The drawing under review shows one solid part. Ordinate dimensions are in mm from its lowest x, y, z. A direction names the side the tool comes from. Coordinates: 2 decimals unless noted, no trailing zeros. Write each loop counter-clockwise with the first axis right and the second up, starting at its lowest first coordinate (ties: lowest second). Pieces come first, ordered by that corner, then holes. Notation, with made-up numbers: (77, 23) - (126, 23) arc R30 cw to (126, 45) - close; hole circle Ø6 at (1.25, -24). An arc over 180 degrees is marked (long way). Use a Markdown table: item, result.
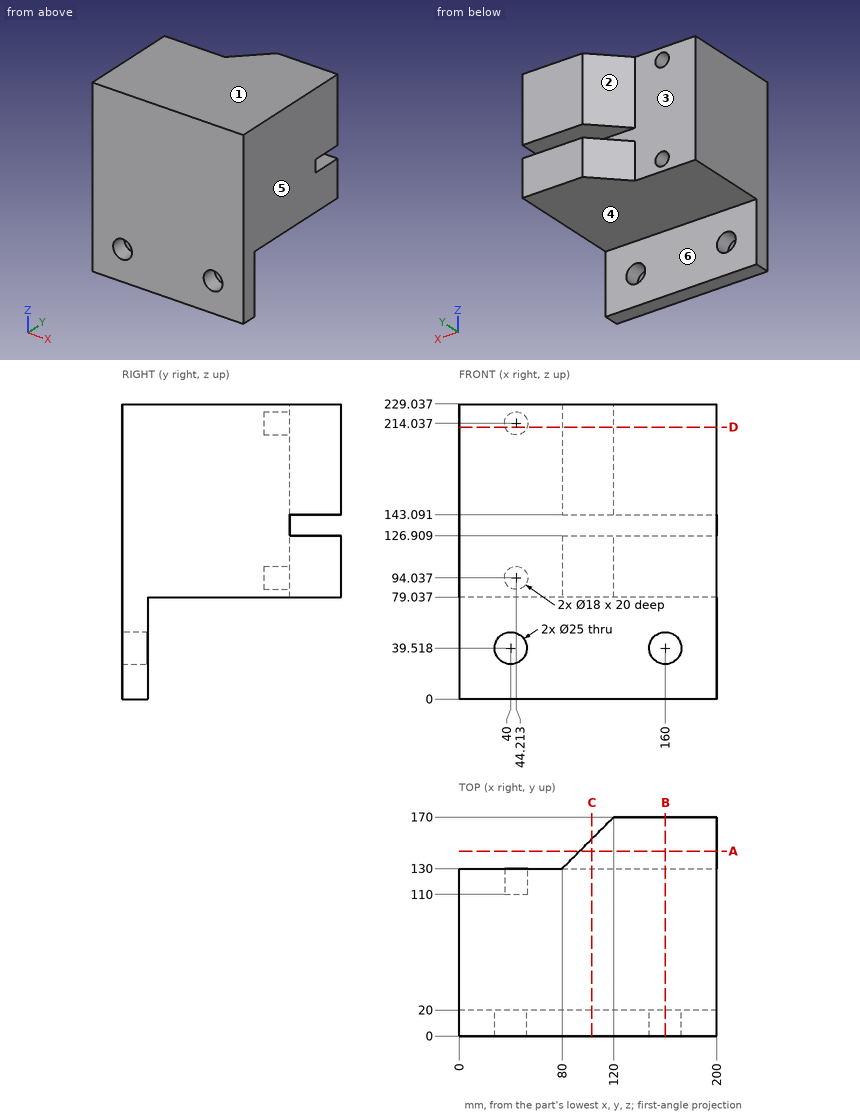
(1) For L1, parallel to Y at x = 80, z = 88; L2, parallel to Y at x = 142, z = 74; L3, parallel to Z at x = 84.5, y = 48, list the stretches that pass through material, from the lowest coordinate up. Write a range as from..to.
Determined:
| item | result |
|---|---|
| L1 | 0..130 |
| L2 | 0..20 |
| L3 | 79.04..229.04 |
(2) Take a section at C-C on x = 103. Write out the cut boundary in (y, z).
Determined:
| item | result |
|---|---|
| outline | (0, 0) - (20, 0) - (20, 79.04) - (153, 79.04) - (153, 126.91) - (130, 126.91) - (130, 143.09) - (153, 143.09) - (153, 229.04) - (0, 229.04) - close |
(3) Draft analysis for pull direction Z (two halves, no side actions). For the marked faces 1, 2, 3 and 4, state which applies: +Z half, -Z half, draft (parallel to the pull), parting line (faces both ways), or undercut.
Determined:
| item | result |
|---|---|
| face 1 | +Z half |
| face 2 | draft |
| face 3 | undercut |
| face 4 | -Z half |
(4) For pin 1 (2 mm diameter, centred on x = 29, z = 122, fed in from +Y); pin 2 (5 mm diameter, centred on x = 60.5, z = 101, fed in from -Y); pin 3 (10 mm diameter, centred on x = 64, y = 77.5, fed in from -Z); pin 4 (9 mm diameter, centred on x = 43, z = 92, fed in from +Y), all flat-tipped, find the tip position at first contact; note any pin that passes through.
Determined:
| item | result |
|---|---|
| pin 1 | y = 130 |
| pin 2 | y = 0 |
| pin 3 | z = 79.04 |
| pin 4 | y = 110 |
(5) Machinability: for the marked faces 5 and 6, which of the approach directions +Z, -Z, +X, -X, +Y, -Y give a long, thin tool a straight path to every point of the face, cutting with its end or side? Answer none if there is none.
Determined:
| item | result |
|---|---|
| face 5 | +Z, -Z, +X, +Y, -Y |
| face 6 | -Z, +X, -X, +Y |
(6) Take a section at B-B on x = 160. Write out the cut boundary in (y, z).
Determined:
| item | result |
|---|---|
| outline | (0, 0) - (20, 0) - (20, 27.02) - (0, 27.02) - close; (0, 52.02) - (20, 52.02) - (20, 79.04) - (170, 79.04) - (170, 126.91) - (130, 126.91) - (130, 143.09) - (170, 143.09) - (170, 229.04) - (0, 229.04) - close |
(7) Take a section at A-A on y = 143.5. Write out the cut boundary in (x, z).
Determined:
| item | result |
|---|---|
| outline | (93.5, 79.04) - (200, 79.04) - (200, 126.91) - (93.5, 126.91) - close; (93.5, 143.09) - (200, 143.09) - (200, 229.04) - (93.5, 229.04) - close |
(8) Take a section at D-D on z = 211. Write out the cut boundary in (x, y) (1 decimal).
Determined:
| item | result |
|---|---|
| outline | (0, 0) - (200, 0) - (200, 170) - (120, 170) - (80, 130) - (52.7, 130) - (52.7, 110) - (35.7, 110) - (35.7, 130) - (0, 130) - close |
